Geometry: see drawing. Coordinates: mm, zero at the bounding-box minimum. A direction names the side the tool comes from. Coordinates: 2 decimals unless noted, no trailing zeros. Loops run counter-clockwise (first coordinate to the right, second up) from the corner with the lowest first, then second, coordinate; pieces in that order, holes last. Notation, with made-up numbers: (66, -6) -> (73, -6) arc R33 cw to (73, 23) -> close; hole circle Ø11 at (46, 21.25). An arc over 180 degrees is marked (long way). One line per question, with ' | ' between items. Start each with the question number.
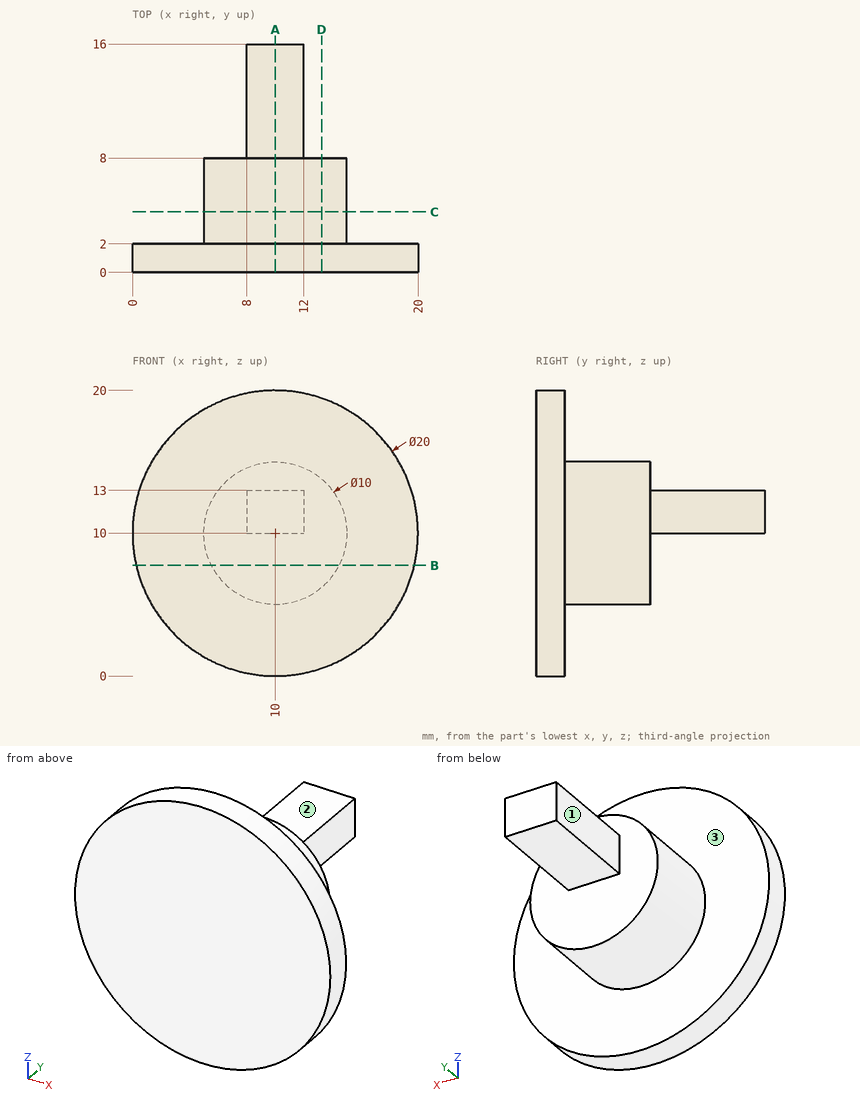
(1) Cut plane C-C, the plane y = 4.25. Return the cut outline in (x, z), and give its area (3 significant figures).
(2) Cut plane A-A, the plane x = 10. Return the cut outline in (y, z), and give its area (3 significant figures).
(3) Ray query, L1, parallel to Y at x = 10.25, z = 14.5; L2, parallel to Y at x = 2, z = 12.25; L3, parallel to Z at x = 9.25, y = 8.25. Return the intervals inside material, ascending.
(4) Cut plane B-B, the plane z = 7.75. Return the cut outline in (x, y).
(5) Access query for the marked faces 1, 2 and 3. Directions: +Z, -Z, +X, -X, +Y, -Y. A direction counts if a zero-diameter tool reaches every point of the face in a straight line with its end or side. Return the directions, or none.
(6) Cut plane D-D, the plane x = 13.25. Return the cut outline in (y, z).
(7) Contact query for flat-ended pins moving along their axis: pin 1 Ø1.5 at (x, y) = (10, 7) entering from +Z; pin 2 Ø5 at (y, z) = (2, 7) entering from -X; pin 3 Ø1.5 at (y, z) = (10, 12) entering from +X. Output: stop coordinate, or through.
Here are the results:
1) outline: circle Ø10 at (10, 10) | area: 78.5 mm2
2) outline: (0, 0) -> (2, 0) -> (2, 5) -> (8, 5) -> (8, 10) -> (16, 10) -> (16, 13) -> (8, 13) -> (8, 15) -> (2, 15) -> (2, 20) -> (0, 20) -> close | area: 124 mm2
3) L1: y = 0 to 8 | L2: y = 0 to 2 | L3: z = 10 to 13
4) outline: (0.26, 0) -> (19.74, 0) -> (19.74, 2) -> (14.47, 2) -> (14.47, 8) -> (5.53, 8) -> (5.53, 2) -> (0.26, 2) -> close
5) face 1: +Z, -Z, -X, +Y | face 2: +Z, +X, -X, +Y | face 3: +Y
6) outline: (0, 0.54) -> (2, 0.54) -> (2, 6.2) -> (8, 6.2) -> (8, 13.8) -> (2, 13.8) -> (2, 19.46) -> (0, 19.46) -> close
7) pin 1: stops at z = 15 | pin 2: stops at x = 0.01 | pin 3: stops at x = 12
